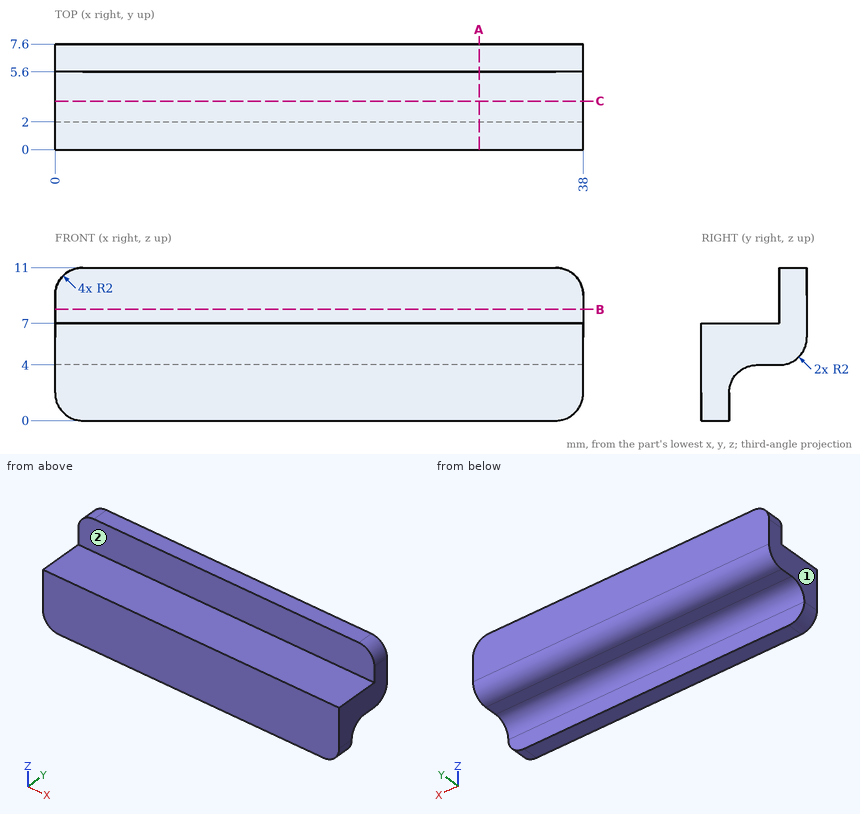
For this review, use the dimensioned drawing (mm, ordinates from the lowest corner) and the shaded views. A direction names the side the tool comes from. Give positions to 0.01 mm unless a question says otherwise; leave off trailing zeros. Write each loop counter-clockwise with the first axis right and the second up, starting at its lowest first coordinate (ties: lowest second). Pieces come first, ordered by that corner, then holes. Notation, with made-up numbers: M 67.25,38.5 L 117.25,38.5 A19 ccw 117.25,49.5 Z; hole C 72.25,86 d5. An arc over 180 degrees is marked long. Answer as a JSON object with one key per item and string values. Group by question number.
Item 1: Consider section A-A on x = 30.5. Write out the cut boundary in (y, z), plus the area to 3 significant figures.
Item 2: For probe 1 along Z at (x, y) = (12.5, 4.75); probe 2 along Y at (x, z) = (35.5, 8.5); probe 3 along Y at (x, z) = (7, 1.25), list the stretches that pass through material, from the lowest coordinate up. Write a range as [from, to].
Item 3: For pin 1 Ø2 at (x, z) = (4, 3.5) entering from +Y; pin 2 Ø3 at (x, y) = (33, 3.5) entering from +Z; pin 3 Ø2 at (x, z) = (23, 4.5) entering from +Y, all flat-tipped, find the tip position at first contact; note any pin that passes through.
Item 4: Consider section B-B on z = 8. Write out the cut boundary in (x, y).
Item 5: Consider section C-C on y = 3.5. Write out the cut boundary in (x, z), plus the area to 3 significant figures.
Item 6: Tool access review of the marked faces 1 and 2: name each direction out of +Z, -Z, +X, -X, +Y, -Y from which nothing blocks a thin tool from reaching the whole face with its end or side.
Check result:
{
 "1": {"outline": "M 0,0 L 2,0 L 2,2 A2 cw 4,4 L 5.6,4 A2 ccw 7.6,6 L 7.6,11 L 5.6,11 L 5.6,7 L 0,7 Z", "area": "38.8 mm^2"},
 "2": {"probe 1": "z = [4, 7]", "probe 2": "y = [5.6, 7.6]", "probe 3": "y = [0, 2]"},
 "3": {"pin 1": "stops at y = 6.92", "pin 2": "stops at z = 7", "pin 3": "stops at y = 7.54"},
 "4": {"outline": "M 0,5.6 L 38,5.6 L 38,7.6 L 0,7.6 Z"},
 "5": {"outline": "M 0,3.94 L 38,3.94 L 38,7 L 0,7 Z", "area": "116 mm^2"},
 "6": {"face 1": "+Z, -Z, -X, +Y, -Y", "face 2": "+Z, +X, -X, -Y"}
}
